from build123d import *

# Parameters (mm, degrees)
SKETCH2_R           = 1.25
BOSS_EXTRUDE1_DEPTH = 3.3
BOSS_EXTRUDE2_DEPTH = 8
SKETCH4_R           = 1.25
CUT_EXTRUDE1_DEPTH  = 4.8
SKETCH5_OUTSIDE_W   = 33.746
SKETCH5_OUTSIDE_H   = 34.442
SKETCH5_OUTSIDE_R   = 2.25
CUT_EXTRUDE2_DEPTH  = 12.3
CUT_EXTRUDE2_TAPER  = 45
SKETCH6_OUTSIDE_W   = 27.146
SKETCH6_OUTSIDE_H   = 27.842
SKETCH6_OUTSIDE_R   = 2.25
CUT_EXTRUDE3_DEPTH  = 9
CUT_EXTRUDE3_TAPER  = 45
CHAMFER1_SIZE       = 0.3


with BuildPart() as part:
    # Sketch2 → Boss-Extrude1 (new body)
    with BuildSketch(Plane.XY):
        Circle(SKETCH2_R)
    extrude(amount=BOSS_EXTRUDE1_DEPTH)

    # Sketch3 → Boss-Extrude2 (add)
    with BuildSketch(Plane(origin=(0, 0, 0), x_dir=(-1, 0, 0), z_dir=(0, 0, -1))):
        Polygon((0, 2.598076211), (-2.25, 1.299038106), (-2.25, -1.299038106), (0, -2.598076211), (2.25, -1.299038106), (2.25, 1.299038106), align=None)
    extrude(amount=BOSS_EXTRUDE2_DEPTH)

    # Sketch4 → Cut-Extrude1 (cut)
    with BuildSketch(Plane(origin=(0, 0, -8), x_dir=(-1, 0, 0), z_dir=(0, 0, -1))):
        Circle(SKETCH4_R)
    extrude(amount=-CUT_EXTRUDE1_DEPTH, mode=Mode.SUBTRACT)

    # Sketch5 outside → Cut-Extrude2 (cut, through all)
    with BuildSketch(Plane(origin=(0, 0, -8), x_dir=(-1, 0, 0), z_dir=(0, 0, -1))):
        Rectangle(SKETCH5_OUTSIDE_W, SKETCH5_OUTSIDE_H)
        Circle(SKETCH5_OUTSIDE_R, mode=Mode.SUBTRACT)
    extrude(amount=-CUT_EXTRUDE2_DEPTH, taper=CUT_EXTRUDE2_TAPER, mode=Mode.SUBTRACT)

    # Sketch6 outside → Cut-Extrude3 (cut, through all)
    with BuildSketch(Plane.XY):
        Rectangle(SKETCH6_OUTSIDE_W, SKETCH6_OUTSIDE_H)
        Circle(SKETCH6_OUTSIDE_R, mode=Mode.SUBTRACT)
    extrude(amount=-CUT_EXTRUDE3_DEPTH, taper=CUT_EXTRUDE3_TAPER, mode=Mode.SUBTRACT)

    # Chamfer1
    chamfer1_edges = [part.edges().sort_by_distance(p)[0] for p in [
        (-1.25, 0, 3.3),
    ]]
    chamfer(chamfer1_edges, length=CHAMFER1_SIZE)


solid = part.part
Check sheet for the modelled part. Datum: model origin and axes. Units: mm. A direction names the side the tool comes from. Coordinates: 2 decimals unless noted, no trailing zeros. Write each loop counter-clockwise with the first axis right and the second up, starting at its lowest first coordinate (ties: lowest second). Pieces come first, ordered by that corner, then holes. Notation, with made-up numbers: M -31,31.5 L 22,31.5 A24 cw 22,65.5 Z; hole C -13.5,27 d1. An arc over 180 degrees is marked long. Answer as CSV lines item,"result".
Q1. Cross-section at B-B (z = 0.5). Record the boundary of the cut face in (x, y), then the cut area to 3 significant figures.
Check result:
outline,"C 0,0 d2.5"
area,"4.91 mm^2"
Q2. Set-up check for faces 4 (the face through (2.25, 0, -4)), 5 (the face through (-0.27, -1.22, 1.48)), 6 (the face through (0, 0, -3.2)): record each of +Z, -Z, +X, -X, +Y, -Y from which the full face is reachable in a straight line by a thin tool's end or side.
Check result:
face 4,"+Z, -Z, +X, +Y, -Y"
face 5,"+Z"
face 6,"-Z"
Q3. Mould release check, pull along Y, two halves, no side actions. Record for faces 1 (the face through (2.058, 1.182, -7.877)), 2 (the face through (-1.109, -1.958, -3.944)), 3 (the face through (0.27, -1.22, -5.63)): released by +Y, released by -Y, zero draft, split by the parting line, or undercut.
Check result:
face 1,"released by +Y"
face 2,"released by -Y"
face 3,"undercut"
Q4. Material ranges on probe 1 along Z at (x, y) = (0.4, -0.6); probe 2 along Z at (x, y) = (-0.45, -1.95); probe 3 along X at (y, z) = (0.25, -6.5), recorded low to high. Write a range as from..to.
Check result:
probe 1,"-3.2..3.3"
probe 2,"-8..0"
probe 3,"-2.25..-1.22, 1.22..2.25"
Q5. Cross-section at A-A (z = -4). Record the boundary of the cut face in (x, y).
Check result:
outline,"M -2.25,-1.3 L 0,-2.6 L 2.25,-1.3 L 2.25,1.3 L 0,2.6 L -2.25,1.3 Z; hole C 0,0 d2.5"
Q6. Go/stop test with a flat-tipped pin: pin 1 (1.5 mm diameter, centred on y = 2, z = 0, fed in from -X). Record where the tip stops, or that it passes through.
Check result:
pin 1,"x = -2.21"
